Input: dimensioned drawing with shaded views. Units: mm. Origin: part minimum x, y, z. Give positions to 0.01 mm unless a question says otherwise; leave off trailing zeros. Write each loop counter-clockwise with the first axis right and the second up, starting at its lowest first coordinate (ties: lowest second). Pieces come first, ordered by that corner, then holes. Notation, with made-up numbers: (49.5, 60.5) -> (87.5, 60.5) arc R18 cw to (87.5, 76.5) -> close; hole circle Ø10 at (29, 30). An arc over 180 degrees is marked (long way). Answer as a JSON object with one key per item and string values.
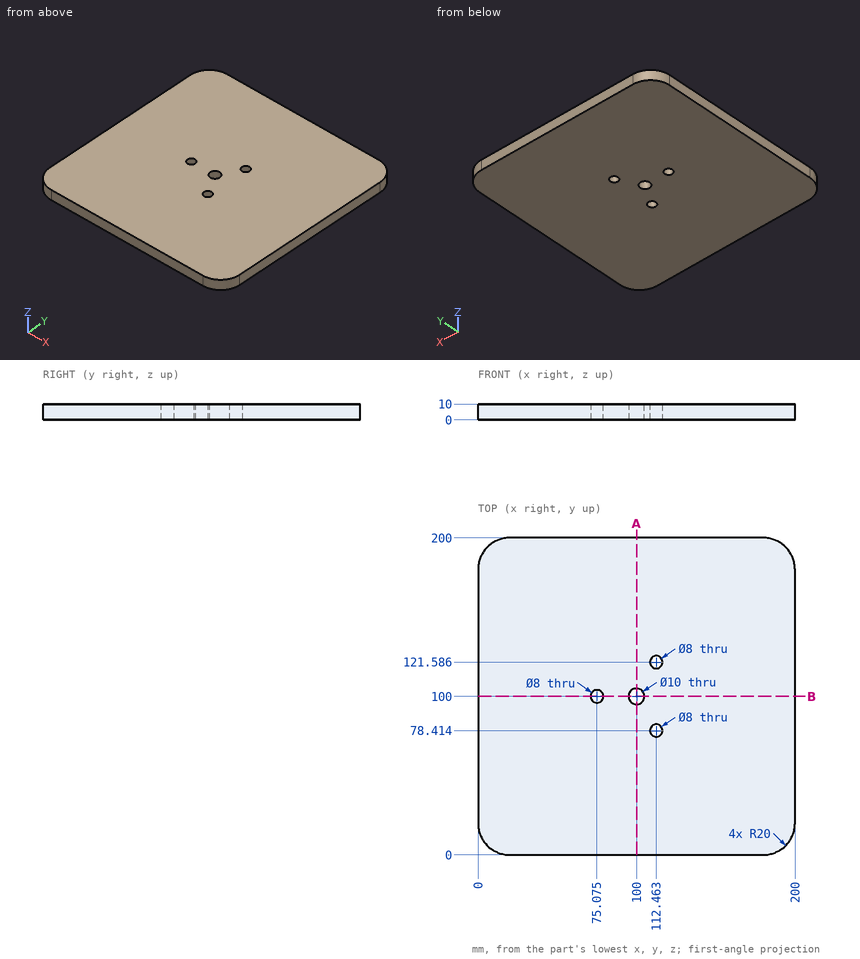
Q1. Cut plane A-A (x = 100). Return the cut outline in (y, z).
Values:
{"outline": "(0, 0) -> (95, 0) -> (95, 10) -> (0, 10) -> close; (105, 0) -> (200, 0) -> (200, 10) -> (105, 10) -> close"}
Q2. Material intervals for L1, parallel to Y at x = 109, z = 0.5 (1 decimal); L2, parallel to Y at x = 109.5, z = 7 (1 decimal); L3, parallel to X at y = 124.5, z = 6.25 (1 decimal), sorted ascending. Write a range as from..to.
Values:
{"L1": "0..76.4, 80.4..119.6, 123.6..200", "L2": "0..75.7, 81.1..118.9, 124.3..200", "L3": "0..109.7, 115.2..200"}
Q3. Cut plane B-B (y = 100). Return the cut outline in (x, z) (1 decimal).
Values:
{"outline": "(0, 0) -> (71.1, 0) -> (71.1, 10) -> (0, 10) -> close; (79.1, 0) -> (95, 0) -> (95, 10) -> (79.1, 10) -> close; (105, 0) -> (200, 0) -> (200, 10) -> (105, 10) -> close"}
Q4. First-contact query: P1, Ø5, axis at y = 54.5, z = 5, coming from the -X side; P2, Ø7, axis at x = 112.46, y = 121.59, coming from the -Z side. Flat tips, straight axial feed; report the tip coordinate or a pass-through.
Values:
{"P1": "x = 0", "P2": "through"}
